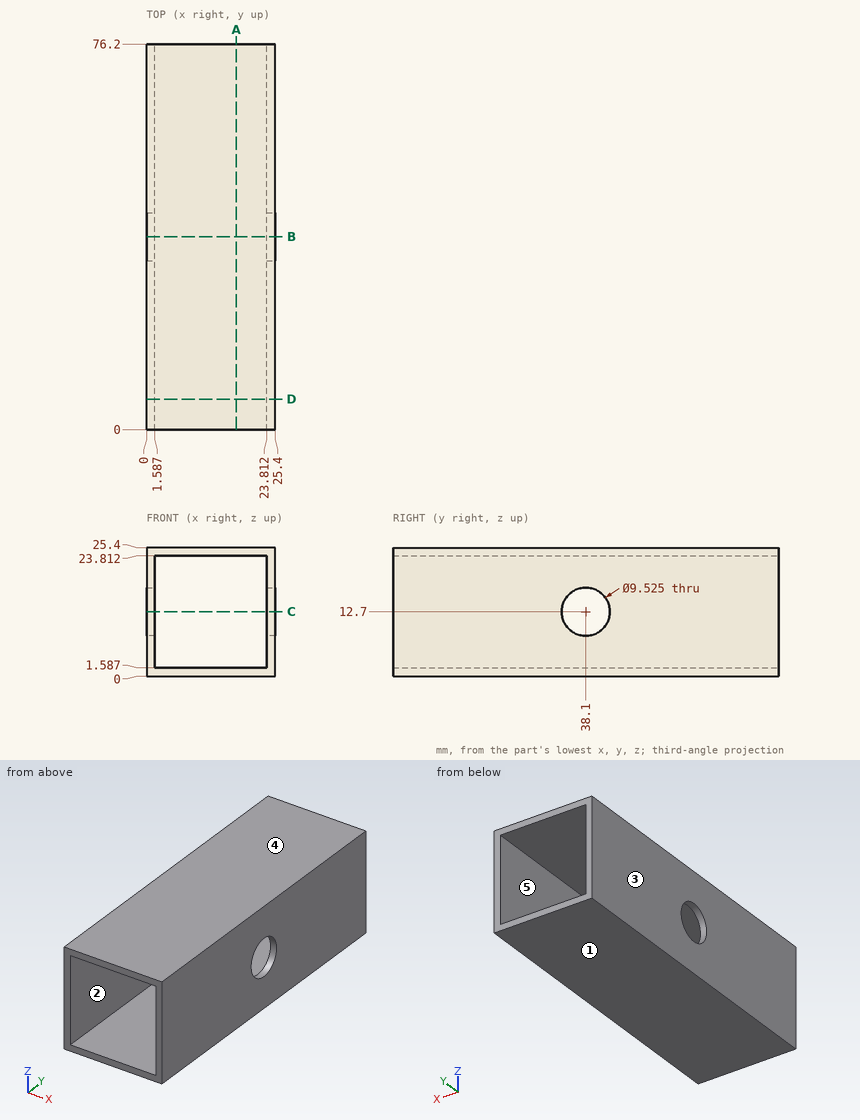
Answer from the drawing. Dimensions are ordinates in mm from the lowest x, y and z of the part. A direction names the side the tool comes from. Give positions to 0.01 mm unless a question says otherwise; leave off trailing zeros. Loops run counter-clockwise (first coordinate to the right, second up) from the corner with the lowest first, then second, coordinate; pieces in that order, holes last.
Item 1: This flat-tipped pin is pushed along its axis until it touches: pin 1 Ø8 at (x, y) = (6, 27) entering from -Z. Where does it stop, or does it pass through?
Derived:
pin 1: stops at z = 0
Item 2: A cutting plane is placed at B-B (y = 38.1). Give the vertices of the cut face in (x, z), then the cut area to 3 significant figures.
Derived:
outline: (0, 0) - (25.4, 0) - (25.4, 7.94) - (23.81, 7.94) - (23.81, 1.59) - (1.59, 1.59) - (1.59, 7.94) - (0, 7.94) - close; (0, 17.46) - (1.59, 17.46) - (1.59, 23.81) - (23.81, 23.81) - (23.81, 17.46) - (25.4, 17.46) - (25.4, 25.4) - (0, 25.4) - close
area: 121 mm2
Item 3: Determine the mould class of the marked faces 1, 2 and 3 for opening direction Z: +Z half, -Z half, draft (parallel to the pull), parting line (faces both ways), or undercut.
Derived:
face 1: -Z half
face 2: undercut
face 3: draft
Item 4: A cutting plane is placed at A-A (x = 17.75). Give the vertices of the cut face in (y, z), then the cut area to 3 significant figures.
Derived:
outline: (0, 0) - (76.2, 0) - (76.2, 1.59) - (0, 1.59) - close; (0, 23.81) - (76.2, 23.81) - (76.2, 25.4) - (0, 25.4) - close
area: 242 mm2
Item 5: A cutting plane is placed at D-D (y = 6). Give the vertices of the cut face in (x, z).
Derived:
outline: (0, 0) - (25.4, 0) - (25.4, 25.4) - (0, 25.4) - close; hole (1.59, 1.59) - (23.81, 1.59) - (23.81, 23.81) - (1.59, 23.81) - close
Item 6: A cutting plane is placed at C-C (z = 12.7). Give the vertices of the cut face in (x, y).
Derived:
outline: (0, 0) - (1.59, 0) - (1.59, 33.34) - (0, 33.34) - close; (0, 42.86) - (1.59, 42.86) - (1.59, 76.2) - (0, 76.2) - close; (23.81, 0) - (25.4, 0) - (25.4, 33.34) - (23.81, 33.34) - close; (23.81, 42.86) - (25.4, 42.86) - (25.4, 76.2) - (23.81, 76.2) - close
Item 7: Find the intervals of material crossed by line 1 along Y through (x, z) = (24.85, 12.7); line 2 along Z through (x, y) = (24.9, 38.1); line 3 along X through (y, z) = (43.5, 7.25), in increasing order.
Derived:
line 1: y = 0 to 33.34, 42.86 to 76.2
line 2: z = 0 to 7.94, 17.46 to 25.4
line 3: x = 0 to 1.59, 23.81 to 25.4
Item 8: A tool of negligible diameter and unlimited length cuts with its end or side. For the marked faces 4 and 5, from which of +Z, -Z, +X, -X, +Y, -Y can it reach the whole face along a straight path? Write none if from no direction.
Derived:
face 4: +Z, +X, -X, +Y, -Y
face 5: +Y, -Y
